from build123d import *

# Parameters (mm, degrees)
SKETCH1_W           = 20
SKETCH1_H           = 120
SKETCH1_R           = 6
BOSS_EXTRUDE2_DEPTH = 20
SKETCH11_R          = 1
CUT_EXTRUDE2_DEPTH  = 21
SKETCH12_R          = 2
CUT_EXTRUDE3_DEPTH  = 5
SKETCH11_3_R        = 1
CUT_EXTRUDE4_DEPTH  = 21
SKETCH14_W          = 20
SKETCH14_H          = 5
SKETCH14_H_2        = 20
CUT_EXTRUDE6_DEPTH  = 2
SKETCH15_W          = 18
SKETCH15_H          = 5
CUT_EXTRUDE7_DEPTH  = 21
SKETCH16_W          = 20
SKETCH16_H          = 12.5
CUT_EXTRUDE8_DEPTH  = 21


with BuildPart() as part:
    # Sketch1 → Boss-Extrude2 (new body)
    with BuildSketch(Plane(origin=(0, 0, 0), x_dir=(0, 0, -1), z_dir=(1, 0, 0))):
        with Locations((10, 60)):
            Rectangle(SKETCH1_W, SKETCH1_H)
        with Locations((10, 82.5)):
            Circle(SKETCH1_R, mode=Mode.SUBTRACT)
    extrude(amount=-BOSS_EXTRUDE2_DEPTH)

    # Sketch11 → Cut-Extrude2 (cut, through all)
    with BuildSketch(Plane.XY):
        with Locations((-15, 10)):
            Circle(SKETCH11_R)
        with Locations((-5, 10)):
            Circle(SKETCH11_R)
    extrude(amount=-CUT_EXTRUDE2_DEPTH, mode=Mode.SUBTRACT)

    # Sketch12 → Cut-Extrude3 (cut)
    with BuildSketch(Plane.XY):
        with Locations((-15, 10)):
            Circle(SKETCH12_R)
        with Locations((-5, 10)):
            Circle(SKETCH12_R)
        with Locations((-15, 100)):
            Circle(SKETCH12_R)
        with Locations((-5, 100)):
            Circle(SKETCH12_R)
    extrude(amount=-CUT_EXTRUDE3_DEPTH, mode=Mode.SUBTRACT)

    # Sketch11<3> → Cut-Extrude4 (cut, through all)
    with BuildSketch(Plane.XY):
        with Locations((-15, 100)):
            Circle(SKETCH11_3_R)
        with Locations((-5, 100)):
            Circle(SKETCH11_3_R)
    extrude(amount=-CUT_EXTRUDE4_DEPTH, mode=Mode.SUBTRACT)

    # Sketch14 → Cut-Extrude6 (cut)
    with BuildSketch(Plane(origin=(0, 0, -20), x_dir=(-1, 0, 0), z_dir=(0, 0, -1))):
        with Locations((10, 100)):
            Rectangle(SKETCH14_W, SKETCH14_H)
        with Locations((10, 10)):
            Rectangle(SKETCH14_W, SKETCH14_H_2)
    extrude(amount=-CUT_EXTRUDE6_DEPTH, mode=Mode.SUBTRACT)

    # Sketch15 → Cut-Extrude7 (cut, through all)
    with BuildSketch(Plane(origin=(0, 0, 0), x_dir=(0, 0, -1), z_dir=(1, 0, 0))):
        with Locations((9, 2.5)):
            Rectangle(SKETCH15_W, SKETCH15_H)
    extrude(amount=-CUT_EXTRUDE7_DEPTH, mode=Mode.SUBTRACT)

    # Sketch16 → Cut-Extrude8 (cut, through all)
    with BuildSketch(Plane(origin=(0, 0, -20), x_dir=(-1, 0, 0), z_dir=(0, 0, -1))):
        with Locations((10, 113.75)):
            Rectangle(SKETCH16_W, SKETCH16_H)
    extrude(amount=-CUT_EXTRUDE8_DEPTH, mode=Mode.SUBTRACT)


solid = part.part
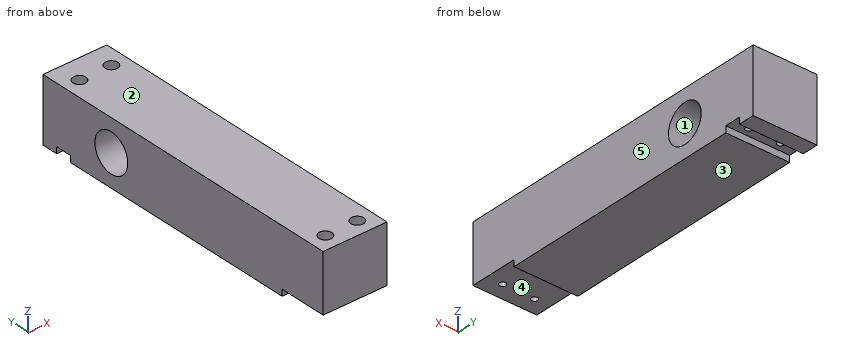
Model file for the job. Use its own axes, mm. Face numbers are marked on the shaded views. A direction names the side the tool comes from. Coordinates: 2 decimals unless noted, no trailing zeros. Write each loop counter-clockwise with the first axis right and the second up, starting at its lowest first coordinate (ties: lowest second). Pieces come first, ordered by that corner, then holes. Notation, with made-up numbers: (27.25, 56) - (36.25, 56) arc R18 ccw to (36.25, 74) - close; hole circle Ø8 at (54, -27.75). An arc over 180 degrees is marked (long way). Write each question's results on one line, items separated by ' | '. Start each with the question number.
1) 3-axis set-ups, long thin cutter, end or side, ignore diameter. For the marked faces 4 and 5: which of +Z, -Z, +X, -X, +Y, -Y reach the whole face in a straight line?
2) Mould opens along Z. For the marked faces 1, 2 and 3 say: pulls with the +Z half, pulls with the -Z half, needs draft (parallel to the pull), parting line crosses it, or undercut.
3) Cut at D-D (y = 10). Write the cut outline in (x, z).
4) Flat gauge pins, fed straight in: P1, Ø1.8, axis at x = -5, y = 100, coming from the +Z side; P2, Ø2, axis at x = -4.5, y = 100.5, coming from the +Z side; P3, Ø12, axis at x = -11, y = 13.5, coming from the -Z side. Where does each tip first touch, or does it go through?
5) Cut at B-B (z = -10). Write the cut outline in (x, y).
6) Cut at C-C (y = 82.5). Write the cut outline in (x, z), then the cut area to 3 significant figures.
7) Cut at A-A (x = -15). Write the cut outline in (y, z), then the cut area to 3 significant figures.
8) Probe line 1 along Y through (x, z) = (-15, -1.4); line 2 along X through (y, z) = (100, -8.75); line 3 along Y through (x, z) = (-5, -10.5). List the from-to ranges inside material, lowest first. Write a range as from..to.
Returned:
1) face 4: -Z, +X, -X, -Y | face 5: +Z, -Z, +X, +Y, -Y
2) face 1: undercut | face 2: pulls with the +Z half | face 3: pulls with the -Z half
3) outline: (-20, -18) - (-16, -18) - (-16, -5) - (-17, -5) - (-17, 0) - (-20, 0) - close; (-14, -18) - (-6, -18) - (-6, -5) - (-7, -5) - (-7, 0) - (-13, 0) - (-13, -5) - (-14, -5) - close; (-4, -18) - (0, -18) - (0, 0) - (-3, 0) - (-3, -5) - (-4, -5) - close
4) P1: through | P2: z = -5 | P3: z = -18
5) outline: (-20, 5) - (0, 5) - (0, 76.5) - (-20, 76.5) - close; (-20, 88.5) - (0, 88.5) - (0, 107.5) - (-20, 107.5) - close; hole circle Ø2 at (-15, 10); hole circle Ø2 at (-15, 100); hole circle Ø2 at (-5, 10); hole circle Ø2 at (-5, 100)
6) outline: (-20, -20) - (0, -20) - (0, -16) - (-20, -16) - close; (-20, -4) - (0, -4) - (0, 0) - (-20, 0) - close | area: 160 mm^2
7) outline: (5, -18) - (9, -18) - (9, -5) - (8, -5) - (8, 0) - (5, 0) - close; (11, -18) - (20, -18) - (20, -20) - (97.5, -20) - (97.5, -18) - (99, -18) - (99, -5) - (98, -5) - (98, 0) - (12, 0) - (12, -5) - (11, -5) - close; (101, -18) - (102.5, -18) - (102.5, -20) - (107.5, -20) - (107.5, 0) - (102, 0) - (102, -5) - (101, -5) - close; hole circle Ø12 at (82.5, -10) | area: 1,800 mm^2
8) line 1: 5..8, 12..98, 102..107.5 | line 2: -20..-16, -14..-6, -4..0 | line 3: 5..9, 11..76.52, 88.48..99, 101..107.5
